from build123d import *

# Parameters (mm, degrees)
ESQUISSE1_W             = 112
ESQUISSE1_H             = 81
BOSS_EXTRU_1_DEPTH      = 2
ESQUISSE2_R             = 1.5
ENL_V_MAT_EXTRU_1_DEPTH = 10
ESQUISSE3_W             = 9.6
ESQUISSE3_H             = 13.1
ESQUISSE3_H_2           = 23.3
ESQUISSE3_H_3           = 18.2
BOSS_EXTRU_2_DEPTH      = 10


with BuildPart() as part:
    # Esquisse1 → Boss.-Extru.1 (new body)
    with BuildSketch(Plane(origin=(0, 0, 0), x_dir=(1, 0, 0), z_dir=(0, 1, 0))):
        Rectangle(ESQUISSE1_W, ESQUISSE1_H)
    extrude(amount=BOSS_EXTRU_1_DEPTH)

    # Esquisse2 → Enlèv. mat.-Extru.1 (cut)
    with BuildSketch(Plane(origin=(0, 2, 0), x_dir=(1, 0, 0), z_dir=(0, 1, 0))):
        with Locations((-50.4, 34.9)):
            Circle(ESQUISSE2_R)
        with Locations((-50.4, -34.9)):
            Circle(ESQUISSE2_R)
        with Locations((24.2, -34.9)):
            Circle(ESQUISSE2_R)
        with Locations((37.7, 18.1)):
            Circle(ESQUISSE2_R)
    extrude(amount=-ENL_V_MAT_EXTRU_1_DEPTH, mode=Mode.SUBTRACT)

    # Esquisse3 → Boss.-Extru.2 (add)
    with BuildSketch(Plane(origin=(0, 2, -2), x_dir=(1, 0, 0), z_dir=(0, -1, 0))):
        with Locations((47.4, 12.15)):
            Rectangle(ESQUISSE3_W, ESQUISSE3_H)
        with Locations((47.4, -8.15)):
            Rectangle(ESQUISSE3_W, ESQUISSE3_H_2)
        with Locations((47.4, -28.47)):
            Rectangle(ESQUISSE3_W, ESQUISSE3_H)
        with Locations((48.442, 29.9)):
            Rectangle(ESQUISSE3_W, ESQUISSE3_H_3)
    extrude(amount=-BOSS_EXTRU_2_DEPTH)


solid = part.part
Design review of the part built by this model. Coordinates are the model's own, in mm. A direction names the side the tool comes from. Give positions to 0.01 mm unless a question says otherwise; leave off trailing zeros. Loops run counter-clockwise (first coordinate to the right, second up) from the corner with the lowest first, then second, coordinate; pieces in that order, holes last. Notation, with made-up numbers: M 70.5,53 L 100.5,53 A26 ccw 100.5,80 Z; hole C 22,-33.5 d8. An arc over 180 degrees is marked long. Write item = value, one per line.
Q1. To check wall thickness, follow line 1 (Z direction, x = -50.4, y = 1.2); line 2 (X direction, y = 0.5, z = 34.9); line 3 (Z direction, x = 24.2, y = 1.6). State the ranges of each line that lie inside material, in increasing order. Write a range as [from, to].
Output values:
line_1 = [-40.5, -36.4], [-33.4, 33.4], [36.4, 40.5]
line_2 = [-56, -51.9], [-48.9, 22.7], [25.7, 56]
line_3 = [-40.5, 33.4], [36.4, 40.5]
Q2. We need section A-A (y = 7). Give the boundary of the cut face in (x, z).
Output values:
outline = M 42.6,-37.02 L 52.2,-37.02 L 52.2,-23.92 L 42.6,-23.92 Z; M 42.6,-21.8 L 52.2,-21.8 L 52.2,1.5 L 42.6,1.5 Z; M 42.6,3.6 L 52.2,3.6 L 52.2,16.7 L 42.6,16.7 Z; M 43.64,18.8 L 53.24,18.8 L 53.24,37 L 43.64,37 Z
Q3. Draft analysis for pull direction X (two halves, no side actions). For faces 1 (the cylindrical face through (22.7, 1.01, 34.83)), 2 (the flat face through (47, 7, -37.02)), 3 (the flat face through (42.6, 7, -10)), 4 (the flat face through (52.2, 7, 10)), state which applies: +X half, -X half, draft (parallel to the pull), parting line (faces both ways), or undercut.
Output values:
face_1 = undercut
face_2 = draft
face_3 = -X half
face_4 = +X half
Q4. For faces 5 (the flat face through (47, 7, 16.7)), 6 (the flat face through (42.6, 7, -31)), 7 (the flat face through (52.2, 7, -10)), list the 3-axis set-ups (+Z, -Z, +X, -X, +Y, -Y) from which the entire face can be reached by the end or side of a thin tool; tool diameter is ignored.
Output values:
face_5 = +X, -X, +Y
face_6 = +Z, -Z, -X, +Y
face_7 = -Z, +X, +Y
Q5. We need section B-B (x = -50.4). Give the boundary of the cut face in (y, z).
Output values:
outline = M 0,-40.5 L 2,-40.5 L 2,-36.4 L 0,-36.4 Z; M 0,-33.4 L 2,-33.4 L 2,33.4 L 0,33.4 Z; M 0,36.4 L 2,36.4 L 2,40.5 L 0,40.5 Z
Q6. We need section C-C (z = 34.9). Give the boundary of the cut face in (x, y), plus the area to 3 significant figures.
Output values:
outline = M -56,0 L -51.9,0 L -51.9,2 L -56,2 Z; M -48.9,0 L 22.7,0 L 22.7,2 L -48.9,2 Z; M 25.7,0 L 56,0 L 56,2 L 53.24,2 L 53.24,12 L 43.64,12 L 43.64,2 L 25.7,2 Z
area = 308 mm^2
Q7. We need section D-D (x = 24.2). Give the boundary of the cut face in (y, z).
Output values:
outline = M 0,-40.5 L 2,-40.5 L 2,33.4 L 0,33.4 Z; M 0,36.4 L 2,36.4 L 2,40.5 L 0,40.5 Z
Q8. Insertion check: pin 1 (5 mm diameter, centred on y = 5, z = 11.5, fed in from -X); pin 2 (3 mm diameter, centred on x = 50, y = 8.5, fed in from +Z); pin 3 (3 mm diameter, centred on x = 48.5, y = 7, fed in from -Z); pin 4 (4 mm diameter, centred on x = 17.5, z = 32.5, fed in from -Y). Each pin has a flat end and moves straight along its axis. Give the tip position at first contact, or say it passes through.
Output values:
pin_1 = 42.6
pin_2 = 37
pin_3 = -37.02
pin_4 = 0
